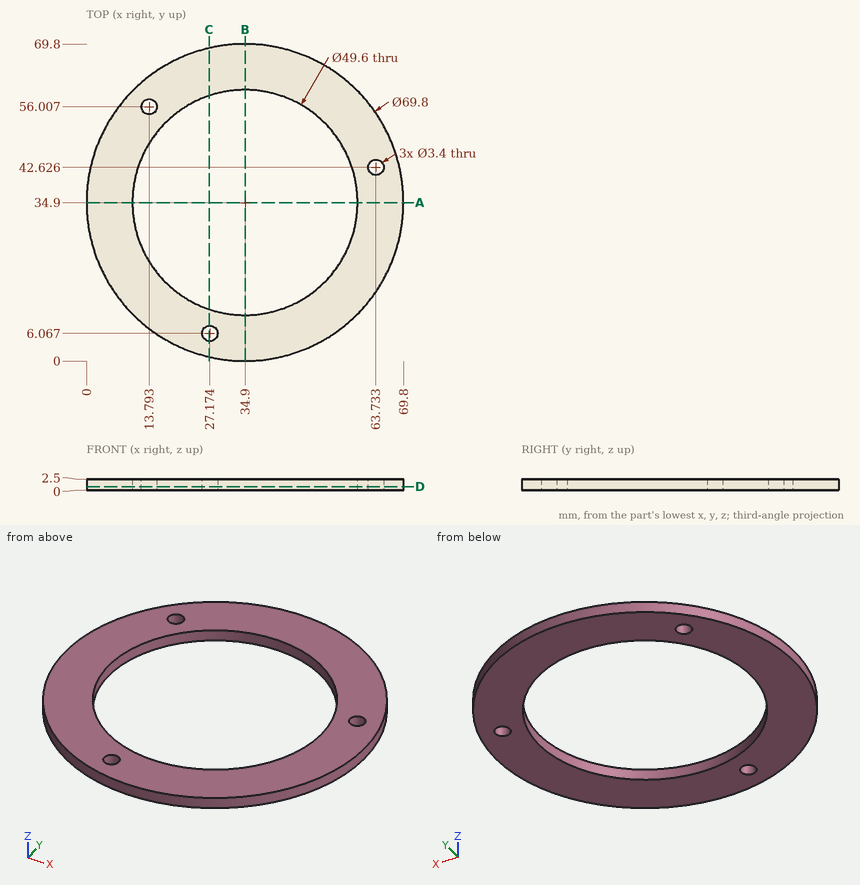
Study the drawing (mm; zero at the part's minimum x, y, z) and answer. Give positions to 0.01 mm unless a question says otherwise; leave off trailing zeros. Loops run counter-clockwise (first coordinate to the right, second up) from the corner with the lowest first, then second, coordinate; pieces in that order, holes last. Notation, with made-up numbers: (48.25, 61) - (95.25, 61) arc R14 cw to (95.25, 72) - close; hole circle Ø4 at (31, 51.25). An arc over 180 degrees is marked (long way). Answer in a Markdown table with one row per item. Add a question column.
Q1. The part is cut by section D-D (z = 0.8). Determine the outline of the cut face in (x, y), and give its area (3 significant figures).
Q2. The part is cut by section C-C (x = 27). Determine the outline of the cut face in (y, z).
Q3. Each of these flat-tipped pins is pushed along its axis until it touches: P1, Ø2.5, axis at x = 63.73, y = 42.63, coming from the -Z side; P2, Ø1.5, axis at x = 37, z = 0.5, coming from the -Y side. Where does it stop, or does it pass through?
Q4. The part is cut by section A-A (y = 34.9). Determine the outline of the cut face in (x, z).
Q5. Consider line 1 along Y through (x, z) = (34.9, 1.65); line 2 along X through (y, z) = (57, 0.3) (1 decimal); line 3 along Y through (x, z) = (19, 2.1). Determine where each line is inside the solid, lowest interval first.
Solution:
| question | item | result |
|---|---|---|
| 1 | outline | circle Ø69.8 at (34.9, 34.9); hole circle Ø49.6 at (34.9, 34.9); hole circle Ø3.4 at (13.79, 56.01); hole circle Ø3.4 at (27.17, 6.07); hole circle Ø3.4 at (63.73, 42.63) |
| 1 | area | 1,870 mm² |
| 2 | outline | (0.91, 0) - (4.38, 0) - (4.38, 2.5) - (0.91, 2.5) - close; (7.76, 0) - (11.39, 0) - (11.39, 2.5) - (7.76, 2.5) - close; (58.41, 0) - (68.89, 0) - (68.89, 2.5) - (58.41, 2.5) - close |
| 3 | P1 | passes through |
| 3 | P2 | stops at y = 0.03 |
| 4 | outline | (0, 0) - (10.1, 0) - (10.1, 2.5) - (0, 2.5) - close; (59.7, 0) - (69.8, 0) - (69.8, 2.5) - (59.7, 2.5) - close |
| 5 | line 1 | y = 0 to 10.1, 59.7 to 69.8 |
| 5 | line 2 | x = 7.9 to 12.4, 15.2 to 23.6, 46.2 to 61.9 |
| 5 | line 3 | y = 3.83 to 15.87, 53.93 to 65.97 |
